Source: three-view drawing plus pictorial views. Frame: mm from the lowest corner of the part. A direction names the side the tool comes from. Give positions to 0.01 mm unless a question says otherwise; leave off trailing zeros. Order: outer loops, then holes, each group sorted by start corner. A loop starts at its lowest first (then second) coordinate and runs counter-clockwise, first axis right, second up.
1) Section D-D, the plane x = 107.5. Return loops of the section in (y, z).
2) Access query for the marked faces 1, 2 and 3. Directions: +Z, -Z, +X, -X, +Y, -Y. A direction counts if a zero-diameter tool reaches every point of the face in a straight line with its end or side. Return the directions, or none.
3) Draft query along X for the marked faces 4, 5, 6 and 7. Return one class per face: released by +X, released by -X, zero draft, split by the parting line, or undercut.
4) First-contact query: P1, Ø12.5, axis at x = 88.5, y = 10, coming from the -Z side; P2, Ø2, axis at x = 101.5, y = 10, coming from the +Z side. Flat tips, straight axial feed; report the tip coordinate or a pass-through.
5) Section A-A, the plane z = 44.5. Return loops of the section in (x, y), plus the area to 3 significant figures.
6) Material intervals for line 1 (X direction, y = 4.75, z = 71); line 2 (Z direction, x = 112.5, y = 7.5); line 3 (Z direction, x = 78, y = 18.5), sorted ascending.
7) Section C-C, the plane x = 86. Return loops of the section in (y, z).
8) Section B-B, the plane y = 16.5. Return loops of the section in (x, z).
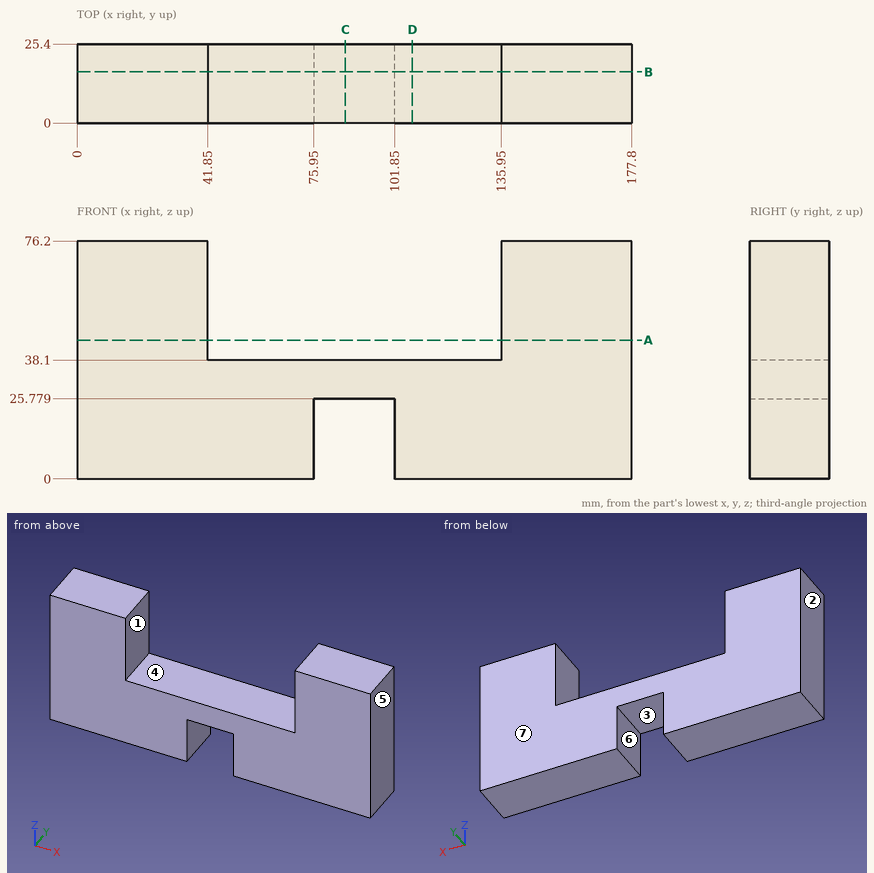
From the geometry:
1. outline: (0, 0) - (25.4, 0) - (25.4, 38.1) - (0, 38.1) - close
2. face 1: +Z, +Y, -Y
2. face 2: +Z, -Z, -X, +Y, -Y
2. face 3: -Z, +Y, -Y
3. face 4: undercut
3. face 5: released by +X
3. face 6: undercut
3. face 7: zero draft
4. P1: stops at z = 25.78
4. P2: stops at z = 38.1
5. outline: (0, 0) - (41.85, 0) - (41.85, 25.4) - (0, 25.4) - close; (135.95, 0) - (177.8, 0) - (177.8, 25.4) - (135.95, 25.4) - close
5. area: 2,130 mm2
6. line 1: x = 0 to 41.85, 135.95 to 177.8
6. line 2: z = 0 to 38.1
6. line 3: z = 25.78 to 38.1
7. outline: (0, 25.78) - (25.4, 25.78) - (25.4, 38.1) - (0, 38.1) - close
8. outline: (0, 0) - (75.95, 0) - (75.95, 25.78) - (101.85, 25.78) - (101.85, 0) - (177.8, 0) - (177.8, 76.2) - (135.95, 76.2) - (135.95, 38.1) - (41.85, 38.1) - (41.85, 76.2) - (0, 76.2) - close
